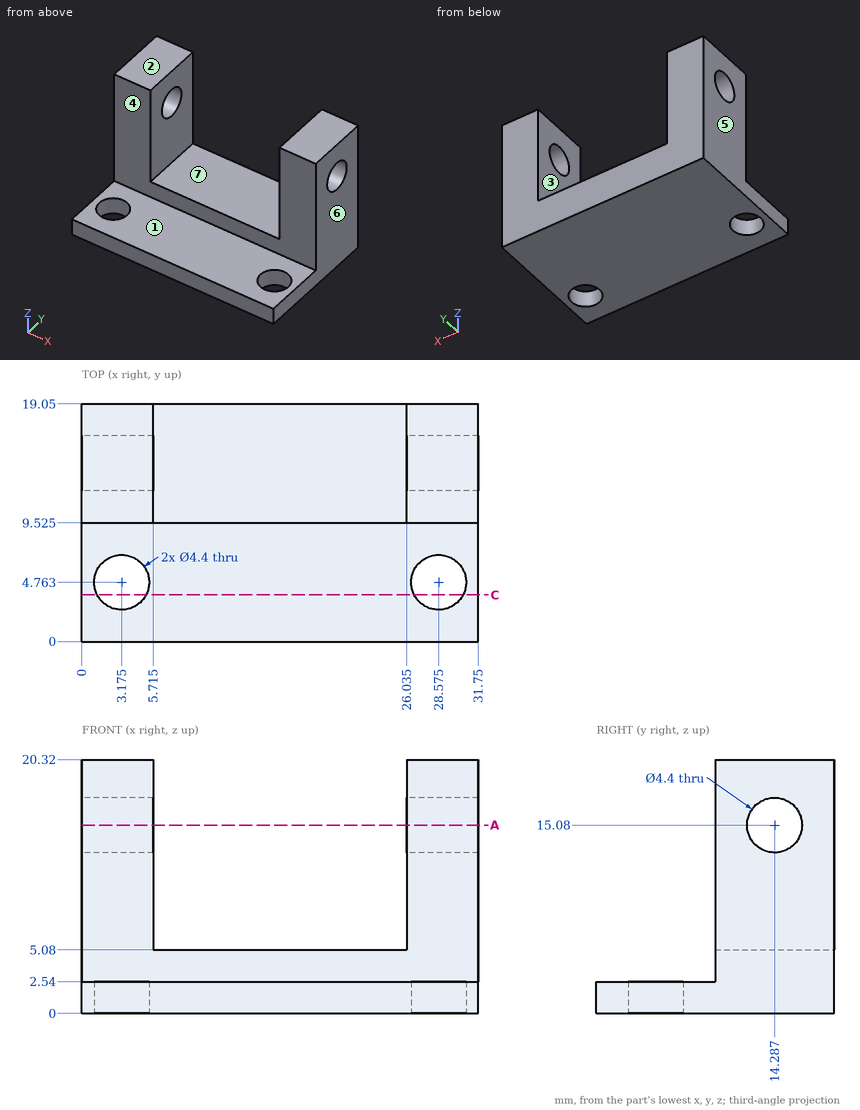
Job drawing, mm, ordinate dimensions from the low corner. One solid piece. A direction names the side the tool comes from. Round coordinates to 2 decimals unless told otherwise and drop trailing zeros. Write each loop counter-clockwise with the first axis right and the second up, starting at its lowest first coordinate (ties: lowest second). Pieces come first, ordered by that corner, then holes. Notation, with made-up numbers: (-6, 34) -> (33, 34) arc R32 cw to (33, 69) -> close; hole circle Ø2 at (11, -3). An arc over 180 degrees is marked (long way). Answer as CSV lines item,"result".
1. Slice it at C-C, the plane y = 3.75. List the corners of the cut face in (x, z).
Resolved:
outline,"(0, 0) -> (1.22, 0) -> (1.22, 2.54) -> (0, 2.54) -> close; (5.13, 0) -> (26.62, 0) -> (26.62, 2.54) -> (5.13, 2.54) -> close; (30.53, 0) -> (31.75, 0) -> (31.75, 2.54) -> (30.53, 2.54) -> close"
2. Slice it at A-A, the plane z = 15.08. State how many separate pieces and enclosed holes the cut face has.
Resolved:
separate pieces,"4"
enclosed holes,"0"
3. Drill centre lines: line 1 (X direction, y = 4, z = 2); line 2 (Z direction, x = 23, y = 15.75); line 3 (Z direction, x = 30.5, y = 14). Where is each one in solid material? Low to high.
Resolved:
line 1,"0 to 1.11, 5.24 to 26.51, 30.64 to 31.75"
line 2,"0 to 5.08"
line 3,"0 to 12.9, 17.26 to 20.32"
4. Pin check, flat tips, straight feed: pin 1 Ø7.5 at (x, y) = (19.5, 16) entering from +Z; pin 2 Ø9 at (x, z) = (11.5, 7.5) entering from -Y (1 decimal); pin 3 Ø8 at (x, y) = (16, 3.5) entering from +Z. Stop position of each tip, or through.
Resolved:
pin 1,"z = 5.08"
pin 2,"y = 9.5"
pin 3,"z = 2.54"
5. Mould opens along X. For the marked faces 4, 5, 6 and 7 say: +X half, -X half, draft (parallel to the pull), parting line (faces both ways), or undercut.
Resolved:
face 4,"draft"
face 5,"-X half"
face 6,"+X half"
face 7,"undercut"
6. Tool access for the marked faces 1, 2 and 3: list every direction of +Z, -Z, +X, -X, +Y, -Y with a clear straight run to the whole face (end or side of a thin tool).
Resolved:
face 1,"+Z, +X, -X, -Y"
face 2,"+Z, +X, -X, +Y, -Y"
face 3,"+Z, +Y, -Y"
